Here's how the part is built. I have some questions about the finished solid (model axes, mm). A direction names the side the tool comes from. Coordinates: 2 decimals unless noted, no trailing zeros. Write each loop counter-clockwise with the first axis right and the second up, starting at its lowest first coordinate (ties: lowest second). Pieces come first, ordered by that corner, then holes. Notation, with made-up numbers: (-13, -22.5) -> (22, -22.5) arc R15 cw to (22, -14.5) -> close; hole circle Ø9 at (4.25, 25). An arc over 180 degrees is marked (long way). Use CSV: the item, a comma, the result in double quotes. Start each with the question number.
```python
from build123d import *

# Parameters (mm, degrees)
SKETCH2_W            = 32.25
SKETCH2_H            = 32.25
BOSS_EXTRUDE1_DEPTH  = 75
SKETCH3_W            = 32.25
SKETCH3_H            = 32.25
BOSS_EXTRUDE2_DEPTH  = 2
SKETCH4_W            = 32.25
SKETCH4_H            = 32.25
BOSS_EXTRUDE3_DEPTH  = 4
FILLET1_R            = 8.75
BOSS_EXTRUDE4_DEPTH  = 32.25
BOSS_EXTRUDE12_DEPTH = 12.5


with BuildPart() as part:
    # Sketch2 → Boss-Extrude1 (new body)
    with BuildSketch(Plane(origin=(0, 0, 0), x_dir=(1, 0, 0), z_dir=(0, 1, 0))):
        Rectangle(SKETCH2_W, SKETCH2_H)
        Polygon((-3.125, 10.125), (-3.125, 3.875), (3.125, 3.875), (3.125, 10.125), (10.125, 10.125), (10.125, 3.125), (3.875, 3.125), (3.875, -3.125), (10.125, -3.125), (10.125, -10.125), (3.125, -10.125), (3.125, -3.875), (-3.125, -3.875), (-3.125, -10.125), (-10.125, -10.125), (-10.125, -3.125), (-3.875, -3.125), (-3.875, 3.125), (-10.125, 3.125), (-10.125, 10.125), align=None, mode=Mode.SUBTRACT)
    extrude(amount=BOSS_EXTRUDE1_DEPTH)

    # Sketch3 → Boss-Extrude2 (add)
    with BuildSketch(Plane.XZ):
        Rectangle(SKETCH3_W, SKETCH3_H)
    extrude(amount=BOSS_EXTRUDE2_DEPTH)

    # Sketch4 → Boss-Extrude3 (add)
    with BuildSketch(Plane.XZ.offset(2)):
        Polygon((-25, 17.5), (-25, 105), (25, 105), (25, 17.5), (55, 17.5), (55, -17.5), (25, -17.5), (25, -105), (-25, -105), (-25, -17.5), (-55, -17.5), (-55, 17.5), align=None)
        Rectangle(SKETCH4_W, SKETCH4_H, mode=Mode.SUBTRACT)
    extrude(amount=-BOSS_EXTRUDE3_DEPTH)

    # Fillet1
    fillet1_edges = [part.edges().sort_by_distance(p)[0] for p in [
        (-25, 0, -105),
        (-25, 0, -17.5),
        (-55, 0, -17.5),
        (-55, 0, 17.5),
        (-25, 0, 17.5),
        (-25, 0, 105),
        (25, 0, 105),
        (25, 0, 17.5),
        (55, 0, 17.5),
        (55, 0, -17.5),
        (25, 0, -17.5),
        (25, 0, -105),
    ]]
    fillet(fillet1_edges, radius=FILLET1_R)

    # Sketch5 → Boss-Extrude4 (add)
    with BuildSketch(Plane(origin=(16.125, 0, 0), x_dir=(0, 0, -1), z_dir=(1, 0, 0))):
        Polygon((16.125, 62), (76.125, 2), (16.125, 2), align=None)
        Polygon((-16.125, 62), (-76.125, 2), (-16.125, 2), align=None)
    extrude(amount=-BOSS_EXTRUDE4_DEPTH)

    # Sketch7 → Boss-Extrude12 (add, symmetric)
    with BuildSketch(Plane.XY):
        Polygon((-16.125, 2), (-46.125, 2), (-16.125, 32), align=None)
        Polygon((46.125, 2), (16.125, 32), (16.125, 2), align=None)
    extrude(amount=BOSS_EXTRUDE12_DEPTH, both=True)


solid = part.part
```
Item 1: I want a section at B-B on x = 13. Please give me the cut outline in (y, z) (3 decimals), then the cut area to 3 significant figures.
Item 2: I want a section at D-D on y = 38. Please give me the cut outline in (x, z) (3 decimals), then the cut area to 3 significant figures.
Item 3: If I drill on line 1 along X through (y, z) = (33, -1.5) (3 decimals); line 2 along X through (y, z) = (25, 8) (3 decimals); line 3 along Y through (x, z) = (-21, 63), over which ranges is the centre line in solid material (lowest first)?
Item 4: I'm going to push flat-ended pins straight in: pin 1 (1.2 mm diameter, centred on y = 0, z = -62, fed in from -X); pin 2 (3 mm diameter, centred on y = 20, z = 35.5, fed in from -X) (3 decimals); pin 3 (10.5 mm diameter, centred on x = 2, y = 67.5, fed in from +Z) (3 decimals). Where does each tip first touch, or does it pass through?
Item 5: Thinking about a two-plate mould opening in X: for faces 1 (the flat face through (25, 0, 62)), 2 (the flat face through (0, 37, -3.875)), 3 (the cylindrical face through (-52.505, 0.028, -14.869)), which applies, +X half, -X half, draft (parallel to the pull), parting line (faces both ways), or undercut?
Item 6: Which directions (+Z, -Z, +X, -X, +Y, -Y) give clear straight access to the entire face, cutting with the end or side of a thin tool? Please do faces 4 (the flat face through (0, 69, 16.125)), 5 (the flat face through (40, 0, -17.5)), 6 (the flat face through (-3.125, 37, 7)).
Item 7: I want a section at C-C on z = 50.5. Please give me the cut outline in (x, y) (3 decimals).
Item 8: I want a section at A-A on y = 65. Please give me the cut outline in (x, z) (3 decimals), then the cut area to 3 significant figures.
Geometry says:
1,outline,"(-2, -105) -> (2, -105) -> (2, -76.125) -> (62, -16.125) -> (75, -16.125) -> (75, 16.125) -> (62, 16.125) -> (2, 76.125) -> (2, 105) -> (-2, 105) -> close"
1,area,"6,790 mm2"
2,outline,"(-16.125, -40.125) -> (16.125, -40.125) -> (16.125, 40.125) -> (-16.125, 40.125) -> close; hole (-10.125, -10.125) -> (-3.125, -10.125) -> (-3.125, -3.875) -> (3.125, -3.875) -> (3.125, -10.125) -> (10.125, -10.125) -> (10.125, -3.125) -> (3.875, -3.125) -> (3.875, 3.125) -> (10.125, 3.125) -> (10.125, 10.125) -> (3.125, 10.125) -> (3.125, 3.875) -> (-3.125, 3.875) -> (-3.125, 10.125) -> (-10.125, 10.125) -> (-10.125, 3.125) -> (-3.875, 3.125) -> (-3.875, -3.125) -> (-10.125, -3.125) -> close"
2,area,"2,330 mm2"
3,line 1,"-16.125 to -3.875, 3.875 to 16.125"
3,line 2,"-23.125 to -10.125, -3.125 to 3.125, 10.125 to 23.125"
3,line 3,"-2 to 2"
4,pin 1,"x = -25"
4,pin 2,"x = -16.125"
4,pin 3,"z = 16.125"
5,face 1,"+X half"
5,face 2,"undercut"
5,face 3,"-X half"
6,face 4,"+Z, +X, -X, +Y"
6,face 5,"-Z, +X, +Y, -Y"
6,face 6,"+Y"
7,outline,"(-25, -2) -> (25, -2) -> (25, 2) -> (16.125, 2) -> (16.125, 27.625) -> (-16.125, 27.625) -> (-16.125, 2) -> (-25, 2) -> close"
8,outline,"(-16.125, -16.125) -> (16.125, -16.125) -> (16.125, 16.125) -> (-16.125, 16.125) -> close; hole (-10.125, -10.125) -> (-3.125, -10.125) -> (-3.125, -3.875) -> (3.125, -3.875) -> (3.125, -10.125) -> (10.125, -10.125) -> (10.125, -3.125) -> (3.875, -3.125) -> (3.875, 3.125) -> (10.125, 3.125) -> (10.125, 10.125) -> (3.125, 10.125) -> (3.125, 3.875) -> (-3.125, 3.875) -> (-3.125, 10.125) -> (-10.125, 10.125) -> (-10.125, 3.125) -> (-3.875, 3.125) -> (-3.875, -3.125) -> (-10.125, -3.125) -> close"
8,area,"786 mm2"
